Here's how the part is built. I have some questions about the finished solid (model axes, mm). A direction names the side the tool comes from. Give positions to 0.01 mm unless a question says otherwise; leave off trailing zeros. Write each loop counter-clockwise with the first axis right and the second up, starting at its lowest first coordinate (ties: lowest second). Pieces come first, ordered by that corner, then holes. Notation, with made-up numbers: (59.25, -25) - (106.25, -25) arc R20 ccw to (106.25, 0) - close; hole circle Ø7 at (-23, 20). An arc over 180 degrees is marked (long way). One line per item, written item: value. Start each with the question number.
1) I'm going to push flat-ended pins straight in: P1, Ø1.5, axis at x = 4.5, y = -10.5, coming from the +Z side; P2, Ø1.2, axis at x = 5, y = 0, coming from the -Z side; P3, Ø0.9, axis at x = 4, z = -12.5, coming from the +Y side. Where does each tip first touch, or does it pass through?
2) We'd pull the mould along Z, two halves only. Please class faces 1 (the flat face through (4, -12, -2)), 2 (the flat face through (4, -2, -12)), 3 (the cylindrical face through (3.96, -9.46, 9.63)): +Z half, -Z half, draft (parallel to the pull), parting line (faces both ways), or undercut.
3) Imagine slicing it at C-C on x = 5.75. Write out the boundary of the cut face in (y, z), plus the area to 3 significant figures.
4) On a 3-axis mill with a long thin cutter (end or side, diameter ignored), from which of +Z, -Z, +X, -X, +Y, -Y can I reach the whole of each face in a straight line? I mean faces 4 (the flat face through (4, 0, -11.5)), 5 (the flat face through (4, -2, 12)), 6 (the flat face through (4, -12, 2)). Say none if no direction works.
5) Imagine slicing it at A-A on y = 0. Write out the boundary of the cut face in (x, z).
6) Please list where these lines run through material, in increasing order: L1, parallel to Y at x = 3.5, z = 0; L2, parallel to Z at x = 1.75, y = 4; L3, parallel to Z at x = 1.25, y = -3.75. Write a range as [from, to].
from build123d import *

# Parameters (mm, degrees)
SKETCH1_R           = 13.5
BOSS_EXTRUDE1_DEPTH = 7
SKETCH2_R           = 7.5
CUT_EXTRUDE1_DEPTH  = 8
CHAMFER1_SIZE       = 1
SKETCH3_W           = 4
SKETCH3_H           = 4
CUT_EXTRUDE2_DEPTH  = 8
CIRPATTERN1_COUNT   = 4


with BuildPart() as part:
    # Sketch1 → Boss-Extrude1 (new body)
    with BuildSketch(Plane(origin=(0, 0, 0), x_dir=(0, 0, -1), z_dir=(1, 0, 0))):
        Circle(SKETCH1_R)
    extrude(amount=BOSS_EXTRUDE1_DEPTH)

    # Sketch2 → Cut-Extrude1 (cut, through all)
    with BuildSketch(Plane(origin=(7, 0, 0), x_dir=(0, 0, -1), z_dir=(1, 0, 0))):
        Circle(SKETCH2_R)
    extrude(amount=-CUT_EXTRUDE1_DEPTH, mode=Mode.SUBTRACT)

    # Chamfer1
    chamfer1_edges = [part.edges().sort_by_distance(p)[0] for p in [
        (0, 0, 13.5),
    ]]
    chamfer(chamfer1_edges, length=CHAMFER1_SIZE)

    # Sketch3 → Cut-Extrude2 (cut, through all)
    with BuildSketch(Plane(origin=(7, 0, 0), x_dir=(0, 0, -1), z_dir=(1, 0, 0))):
        with Locations((0, 13.5)):
            Rectangle(SKETCH3_W, SKETCH3_H)
    cut_extrude2 = extrude(amount=-CUT_EXTRUDE2_DEPTH, mode=Mode.SUBTRACT)

    # CirPattern1: Cut-Extrude2 ×4 about axis
    cirpattern1_axis = Axis((0, 0, 0), (1, 0, 0))
    for i in range(1, CIRPATTERN1_COUNT):
        add(cut_extrude2.rotate(cirpattern1_axis, i * 360 / CIRPATTERN1_COUNT), mode=Mode.SUBTRACT)


solid = part.part
Numbers:
1. P1: z = 9.34
1. P2: z = -11.5
1. P3: y = 6.09
2. face 1: undercut
2. face 2: draft
2. face 3: +Z half
3. outline: (-13.35, -2) arc R13.5 ccw to (-2, -13.35) - (-2, -11.5) - (2, -11.5) - (2, -13.35) arc R13.5 ccw to (13.35, -2) - (11.5, -2) - (11.5, 2) - (13.35, 2) arc R13.5 ccw to (2, 13.35) - (2, 11.5) - (-2, 11.5) - (-2, 13.35) arc R13.5 ccw to (-13.35, 2) - (-11.5, 2) - (-11.5, -2) - close; hole circle Ø15 at (0, 0)
3. area: 365 mm^2
4. face 4: -Z, +X, -X
4. face 5: +Z, +X, -X
4. face 6: +X, -X, -Y
5. outline: (0, -11.5) - (7, -11.5) - (7, -7.5) - (0, -7.5) - close; (0, 7.5) - (7, 7.5) - (7, 11.5) - (0, 11.5) - close
6. L1: [-11.5, -7.5], [7.5, 11.5]
6. L2: [-12.89, -6.34], [6.34, 12.89]
6. L3: [-12.97, -6.5], [6.5, 12.97]
